Autodesk Inventor part; units mm, degrees
ref_plane "YZ Plane" through (0, 0, 0) normal (1, 0, 0) x (0, 1, 0)
ref_plane "XZ Plane" through (0, 0, 0) normal (0, 1, 0) x (-1, 0, 0)
ref_plane "XY Plane" through (0, 0, 0) normal (0, 0, 1) x (1, 0, 0)
sketch "Schizzo1" plane through (0, 0, 0) normal (0, 0, 1) x (1, 0, 0)
  line L0 (40, -40) -> (-40, -40)
  line L1 (-40, -40) -> (-40, 40)
  line L2 (-40, 40) -> (40, 40)
  line L3 (40, 40) -> (40, -40)
  line L4 (40, -40) -> (-40, 40) construction
  line L5 (-40, -40) -> (40, 40) construction
  circle A0 centre (0, 0) radius 22.5
  dimension "d0" = 80
  dimension "d1" = 80
  dimension "d2" = 45
extrude "Estrusione1" add sketch "Schizzo1" along normal mid plane 1.5
fillet "Raccordo1" radius 5 4 edges at (40, 40, 0) (40, -40, 0) (-40, -40, 0) (-40, 40, 0)
sketch "Schizzo2" plane through (0, 0, 0.75) normal (0, 0, 1) x (1, 0, 0)
  line L0 (35, -40) -> (-35, -40)
  line L1 (0, -40) -> (0, -38)
  line L2 (0, -38) -> (35, -38)
  line L3 (0, -38) -> (-35, -38)
  line L4 (-40, -35) -> (-40, 35)
  line L5 (-40, 0) -> (-38, 0)
  line L6 (-38, 0) -> (-38, -35)
  arc A0 (-38, -35) -> (-35, -38) centre (-35, -35) ccw
  line L7 (40, 35) -> (40, -35)
  line L8 (0, 38) -> (35, 38)
  line L9 (0, 38) -> (-35, 38)
  line L10 (-38, 0) -> (-38, 35)
  arc A1 (-35, 38) -> (-38, 35) centre (-35, 35) ccw
  line L11 (35, 40) -> (-35, 40)
  line L12 (38, 0) -> (38, 35)
  arc A2 (38, 35) -> (35, 38) centre (35, 35) ccw
  line L13 (38, 0) -> (38, -35)
  arc A3 (35, -38) -> (38, -35) centre (35, -35) ccw
  circle A4 centre (0, 0) radius 24.5
  dimension "d6" = 2
  dimension "d8" = 35
  dimension "d9" = 35
  dimension "d10" = 2
  dimension "d11" = 35
extrude "Estrusione2" cut sketch "Schizzo2" against normal blind 0.5
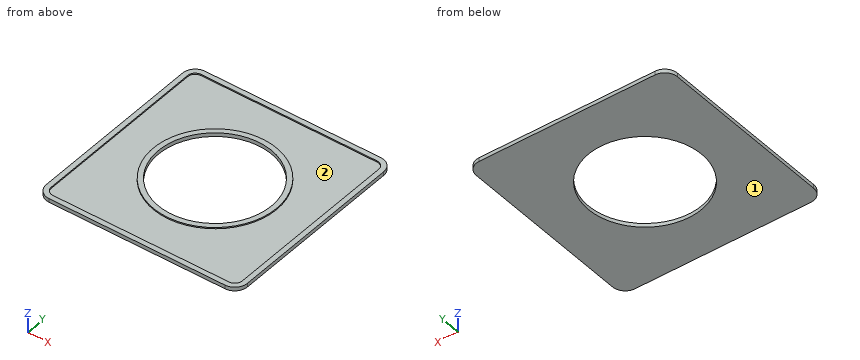
Can you work these out from the model? Positions are in its coordinate system, mm. Face numbers are marked on the shaded views. Coordinates: 2 decimals unless noted, no trailing zeros. Loops run counter-clockwise (first coordinate to the right, second up) from the corner with the lowest first, then second, coordinate; pieces in that order, holes last. Notation, with made-up numbers: M 22.5,-24 L 81.5,-24 A32 ccw 81.5,8 Z; hole C 14,-27 d7. An arc over 180 degrees is marked long. Put each result on its own line as item: value. Start each with the question number.
(1) Imagine slicing it at A-A on y = 0. List the corners of the cut face in (x, z) for me.
(2) Imagine slicing it at C-C on x = 32.5. List the corners of the cut face in (y, z) for me, and give its area (3 significant figures).
(3) We'd pull the mould along Y, two halves only. Please class the marked faces 1 and 2: +Y half, -Y half, draft (parallel to the pull), parting line (faces both ways), or undercut.
(4) I need wall thicknesses on probe 1 along Y at (x, z) = (0, 0.4); probe 2 along Y at (x, z) = (0, 0); probe 3 along X at (y, z) = (25.5, 0.5). Which ranges of each line are inside material? Lowest first, please.
(5) Will these pins go through, and if not, where does the flat tip stop? pin 1 Ø10 at (x, y) = (-11.5, -31) entering from +Z; pin 2 Ø10 at (x, y) = (19.5, -1.5) entering from +Z.
Worked answers:
1. outline: M -40,-0.75 L -22.5,-0.75 L -22.5,0.75 L -24.5,0.75 L -24.5,0.25 L -38,0.25 L -38,0.75 L -40,0.75 Z; M 22.5,-0.75 L 40,-0.75 L 40,0.75 L 38,0.75 L 38,0.25 L 24.5,0.25 L 24.5,0.75 L 22.5,0.75 Z
2. outline: M -40,-0.75 L 40,-0.75 L 40,0.75 L 38,0.75 L 38,0.25 L -38,0.25 L -38,0.75 L -40,0.75 Z
2. area: 82.0 mm2
3. face 1: draft
3. face 2: undercut
4. probe 1: y = -40 to -38, -24.5 to -22.5, 22.5 to 24.5, 38 to 40
4. probe 2: y = -40 to -22.5, 22.5 to 40
4. probe 3: x = -40 to -38, 38 to 40
5. pin 1: stops at z = 0.25
5. pin 2: stops at z = 0.75
